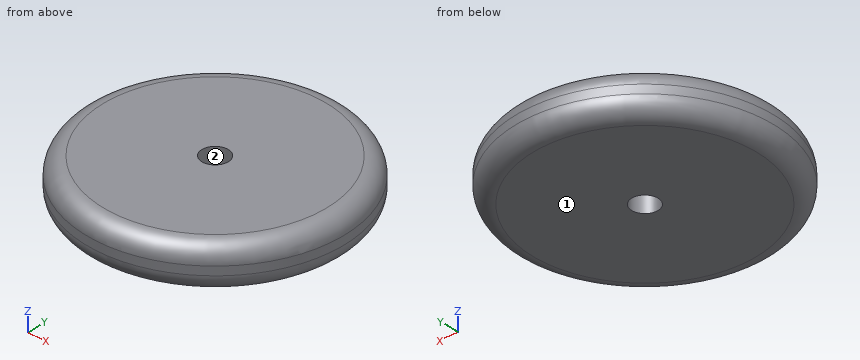
```python
from build123d import *

# Parameters (mm, degrees)
F0_R     = 11.43
F1_DEPTH = 1.905
F2_R     = 1.1684
F3_DEPTH = 25.4
F4_R     = 1.524


with BuildPart() as f1:
    # F0 (on Top) → F1 (new body, symmetric)
    with BuildSketch(Plane.XY):
        Circle(F0_R)
    extrude(amount=F1_DEPTH, both=True)

    # F2 (on face) → F3 (cut)
    with BuildSketch(Plane(origin=(0, 0, -1.905), x_dir=(1, 0, 0), z_dir=(0, 0, -1))):
        Circle(F2_R)
    extrude(amount=-F3_DEPTH, mode=Mode.SUBTRACT)

    # F4
    f4_edges = [f1.edges().sort_by_distance(p)[0] for p in [
        (-11.43, 0, 1.905),
        (-11.43, 0, -1.905),
    ]]
    fillet(f4_edges, radius=F4_R)


solid = f1.part
```
Input: part model. Units: mm. Frame: model coordinates. Face numbers are marked on the shaded views. Give positions to 0.01 mm unless a question says otherwise; leave off trailing zeros. Order: outer loops, then holes, each group sorted by start corner. A loop starts at its lowest first (then second) coordinate and runs counter-clockwise, first axis right, second up. Notation, with made-up numbers: (-8, -21.75) - (9, -21.75) arc R22 cw to (9, -15.75) - close; hole circle Ø1 at (44, 87.25). An arc over 180 degrees is marked (long way). Use a Markdown table: item, result.
(1) Pin query (flat end, axial travel): pin 1 (1 mm diameter, centred on x = 3.5, z = 0, fed in from +Y); pin 2 (1.5 mm diameter, centred on x = -6, z = 1.5, fed in from +Y); pin 3 (1.4 mm diameter, centred on x = 0, y = 0, fed in from +Z); pin 4 (1 mm diameter, centred on y = 2.5, z = -1, fed in from -X). Return the tip coordinate at first contact, or that it passes through.
Computed values:
| item | result |
|---|---|
| pin 1 | stops at y = 11.03 |
| pin 2 | stops at y = 9.9 |
| pin 3 | passes through |
| pin 4 | stops at x = -11.2 |
(2) Line query: line 1 (Y direction, x = 0, z = 0.4); line 2 (X direction, y = -4.25, z = 0.6); line 3 (X direction, y = -7.25, z = 1.5). Output: solid intervals per line, ascending. Write a range as from..to.
Computed values:
| item | result |
|---|---|
| line 1 | y = -11.43..-1.17, 1.17..11.43 |
| line 2 | x = -10.59..10.59 |
| line 3 | x = -8.19..8.19 |
(3) Section query D-D (z = 1.5). Output: boundary loops of the cut face in (x, y), then the cut area to 3 significant figures.
Computed values:
| item | result |
|---|---|
| outline | circle Ø21.88 at (0, 0); hole circle Ø2.34 at (0, 0) |
| area | 372 mm2 |
(4) Section query A-A (y = 0). Output: boundary loops of the cut face in (x, z) (3 decimals).
Computed values:
| item | result |
|---|---|
| outline | (-11.43, -0.381) arc R1.524 ccw to (-9.906, -1.905) - (-1.168, -1.905) - (-1.168, 1.905) - (-9.906, 1.905) arc R1.524 ccw to (-11.43, 0.381) - close; (1.168, -1.905) - (9.906, -1.905) arc R1.524 ccw to (11.43, -0.381) - (11.43, 0.381) arc R1.524 ccw to (9.906, 1.905) - (1.168, 1.905) - close |
(5) Section query C-C (z = -1.6). Output: boundary loops of the cut face in (x, y), then the cut area to 3 significant figures.
Computed values:
| item | result |
|---|---|
| outline | circle Ø21.64 at (0, 0); hole circle Ø2.34 at (0, 0) |
| area | 364 mm2 |
(6) Draft query along Y for the marked faces 1 and 2. Return one class per face: released by +Y, released by -Y, zero draft, split by the parting line, or undercut.
Computed values:
| item | result |
|---|---|
| face 1 | zero draft |
| face 2 | undercut |
